from build123d import *

# Parameters (mm, degrees)
CROQUIS1_W              = 50
CROQUIS1_H              = 20
SALIENTE_EXTRUIR1_DEPTH = 25
CROQUIS5_W              = 46
CROQUIS5_H              = 20
CORTAR_EXTRUIR1_DEPTH   = 17
SALIENTE_EXTRUIR2_DEPTH = 25
CORTAR_EXTRUIR5_DEPTH   = 24
CHAFL_N2_SIZE           = 10
CHAFL_N2_SIZE_2         = 7.26542528


with BuildPart() as part:
    # Croquis1 → Saliente-Extruir1 (new body)
    with BuildSketch(Plane(origin=(0, 0, 0), x_dir=(1, 0, 0), z_dir=(0, 1, 0))):
        Rectangle(CROQUIS1_W, CROQUIS1_H)
    extrude(amount=SALIENTE_EXTRUIR1_DEPTH)

    # Croquis5 → Cortar-Extruir1 (cut)
    with BuildSketch(Plane(origin=(0, 2.566177554, 10), x_dir=(1, 0, 0), z_dir=(0, 0, 1))):
        with Locations((0.564953321, 8.627432653)):
            Rectangle(CROQUIS5_W, CROQUIS5_H)
    extrude(amount=-CORTAR_EXTRUIR1_DEPTH, mode=Mode.SUBTRACT)

    # Croquis6 → Saliente-Extruir2 (add)
    with BuildSketch(Plane.XZ):
        with BuildLine():
            Line((-22.217043892, -6.976270562), (17.782956108, -6.976270562))
            ThreePointArc((17.782956108, -6.976270562), (-2.217043892, -26.976270562), (-22.217043892, -6.976270562))
        make_face()
    extrude(amount=-SALIENTE_EXTRUIR2_DEPTH)

    # Croquis11 → Cortar-Extruir5 (cut)
    with BuildSketch(Plane(origin=(0, 25, 0), x_dir=(1, 0, 0), z_dir=(0, 1, 0))):
        with BuildLine():
            Line((-20.391864193, 6.892929863), (15.608135807, 6.892929863))
            ThreePointArc((15.608135807, 6.892929863), (-2.391864193, 24.892929863), (-20.391864193, 6.892929863))
        make_face()
    extrude(amount=-CORTAR_EXTRUIR5_DEPTH, mode=Mode.SUBTRACT)

    # Chaflán2
    # the kernel refuses this chamfer: 10, 7.26542528 mm, written as the material it adds along each edge
    with BuildSketch(Plane(origin=(23.564953321, 1.193610207, -7), x_dir=(0.022768510603911864, 0, 0.9997407638607518), z_dir=(0, 1, 0))) as chafl_n2_piece_1:
        Polygon((CHAFL_N2_SIZE * 0.999740763861, -CHAFL_N2_SIZE * 0.0227685106039), (-CHAFL_N2_SIZE_2 * 0.0227685106041, -CHAFL_N2_SIZE_2 * 0.999740763868), (0, 0), align=None)
    extrude(amount=20)
    # the kernel refuses this chamfer: 10, 7.26542528 mm, written as the material it takes off along each edge
    with BuildSketch(Plane(origin=(25, -25.815709359, -10), x_dir=(0.022768510603911864, 0, 0.9997407638607518), z_dir=(0, 1, 0))) as chafl_n2_2_piece_1:
        Polygon((CHAFL_N2_SIZE * 0.999740763861, -CHAFL_N2_SIZE * 0.0227685106039), (-CHAFL_N2_SIZE_2 * 0.0227685106041, -CHAFL_N2_SIZE_2 * 0.999740763868), (0, 0), align=None)
    extrude(amount=76.631418718, mode=Mode.SUBTRACT)


solid = part.part
For this review, take the finished solid that the model builds, in its own axes (mm). A direction names the side the tool comes from. Round coordinates to 2 decimals unless told otherwise and drop trailing zeros. Loops run counter-clockwise (first coordinate to the right, second up) from the corner with the lowest first, then second, coordinate; pieces in that order, holes last. Notation, with made-up numbers: (18.25, 10) - (32.25, 10) arc R33 cw to (32.25, 38) - close; hole circle Ø4 at (1.5, 29). An arc over 180 degrees is marked (long way). Use one line per item in the form item = value.
1) We need section D-D on z = -15.5. Write out the cut boundary in (x, y), then the cut area to 3 significant figures.
Solutions:
outline = (-20.31, 0) - (15.88, 0) - (15.88, 25) - (13.42, 25) - (13.42, 1) - (-18.2, 1) - (-18.2, 25) - (-20.31, 25) - close
area = 146 mm2
2) We need section A-A on y = 21.75. Write out the cut boundary in (x, z), then the cut area to 3 significant figures.
Solutions:
outline = (-25, -10) - (-21.99, -10) arc R20 ccw to (17.55, -10) - (17.73, -10) - (25, 0) - (25, 10) - (-25, 10) - close; hole (-20.39, -6.89) arc R18 ccw to (15.61, -6.89) - close
area = 963 mm2
3) Clearance check with flat-ended pins moving along their axes: P1, Ø2, axis at x = -21, y = 15, coming from the +Z side; P2, Ø1.5, axis at y = 13.5, z = -15.5, coming from the +X side; P3, Ø6, axis at x = 4.5, y = 6.5, coming from the +Z side. State where each tip first meets the part, or that it passes through.
Solutions:
P1 = -6.98
P2 = 16.21
P3 = -21.93
4) We need section B-B on x = -6. Write out the cut boundary in (y, z).
Solutions:
outline = (0, -26.62) - (25, -26.62) - (25, -24.53) - (1, -24.53) - (1, -6.89) - (1.19, -6.89) - (1.19, 10) - (0, 10) - close; (21.19, -6.89) - (25, -6.89) - (25, 10) - (21.19, 10) - close
5) Wall thickness on probe 1 along Y at (x, z) = (-11, -4); probe 2 along Y at (x, z) = (-7.5, -16.5); probe 3 along X at (y, z) = (2.75, 3.5): over which ranges is each line inside the solid? List them lowest first.
Solutions:
probe_1 = 0 to 1.19, 21.19 to 25
probe_2 = 0 to 1
probe_3 = -25 to -22.44, 23.56 to 25
6) Tool access review of faces 4 (the face through (0, 1.194, 2)), 5 (the face through (-25, 12, 0)), 6 (the face through (-3, 1, -14)), 7 (the face through (-24, 12, -10)): name each direction out of +Z, -Z, +X, -X, +Y, -Y from which nothing blocks a thin tool from reaching the whole face with its end or side.
Solutions:
face_4 = +Z
face_5 = +Z, -Z, -X, +Y, -Y
face_6 = +Y
face_7 = -Z, -X, +Y, -Y
7) Mouldability with a two-part tool opening along Z and no side actions: class faces 1 (the face through (-3, 23, -6.893)), 2 (the face through (-21, 11, -6.976)), 3 (the face through (21.42, 12.33, -4.93)) as pulls with the +Z half, pulls with the -Z half, needs draft (parallel to the pull), parting line crosses it, or undercut.
Solutions:
face_1 = undercut
face_2 = pulls with the +Z half
face_3 = pulls with the -Z half
